```python
from build123d import *

# Parameters (mm, degrees)
SKETCH_1_W                = 38
SKETCH_1_H                = 46.5
EXTRUDE_1_DEPTH           = 7
SKETCH_2_W                = 5
SKETCH_2_H                = 38.5
CUT_EXTRUDE_1_DEPTH       = 52.100391388
SKETCH_3_W                = 7
SKETCH_3_H                = 39.5
CUT_EXTRUDE_2_DEPTH       = 52.100391388
SKETCH_4_W                = 7.5
SKETCH_4_H                = 20
CUT_EXTRUDE_3_DEPTH       = 52.100391388
SKETCH_5_W                = 7.5
SKETCH_5_H                = 20
CUT_EXTRUDE_4_DEPTH       = 52.100391388
SKETCH_6_W                = 26
SKETCH_6_H                = 6
EXTRUDE_2_DEPTH           = 41.75
HOLE_WIZARD_3_0_3_1_D     = 3
HOLE_WIZARD_3_0_3_1_DEPTH = 8
HOLE_WIZARD_3_0_3_2_D     = 3
HOLE_WIZARD_3_0_3_2_DEPTH = 48.75
HOLE_WIZARD_3_0_3_3_D     = 3
HOLE_WIZARD_M201_D        = 22.1
HOLE_WIZARD_M201_DEPTH    = 46.5
FILLET_1_R                = 10


with BuildPart() as part:
    # Эскиз1 → Бобышка-Вытянуть1 (new body)
    with BuildSketch(Plane(origin=(24.375, 0, 0), x_dir=(0, 0, -1), z_dir=(1, 0, 0))):
        with Locations((-1, 23.25)):
            Rectangle(SKETCH_1_W, SKETCH_1_H)
    extrude(amount=-EXTRUDE_1_DEPTH)

    # Эскиз2 → Вырез-Вытянуть1 (cut, through all)
    with BuildSketch(Plane.ZY.offset(-17.375)):
        with Locations((-15.5, 27.25)):
            Rectangle(SKETCH_2_W, SKETCH_2_H)
    extrude(amount=-CUT_EXTRUDE_1_DEPTH, mode=Mode.SUBTRACT)

    # Эскиз3 → Вырез-Вытянуть2 (cut, through all)
    with BuildSketch(Plane.ZY.offset(-17.375)):
        with Locations((16.5, 26.75)):
            Rectangle(SKETCH_3_W, SKETCH_3_H)
    extrude(amount=-CUT_EXTRUDE_2_DEPTH, mode=Mode.SUBTRACT)

    # Эскиз4 → Вырез-Вытянуть3 (cut, through all)
    with BuildSketch(Plane(origin=(24.375, 0, 0), x_dir=(0, 0, -1), z_dir=(1, 0, 0))):
        with Locations((-7.5, 28.5)):
            Rectangle(SKETCH_4_W, SKETCH_4_H)
    extrude(amount=-CUT_EXTRUDE_3_DEPTH, mode=Mode.SUBTRACT)

    # Эскиз5 → Вырез-Вытянуть4 (cut, through all)
    with BuildSketch(Plane.ZY.offset(-17.375)):
        with Locations((-7.5, 28.5)):
            Rectangle(SKETCH_5_W, SKETCH_5_H)
    extrude(amount=-CUT_EXTRUDE_4_DEPTH, mode=Mode.SUBTRACT)

    # Эскиз6 → Бобышка-Вытянуть2 (add)
    with BuildSketch(Plane.ZY.offset(-17.375)):
        with Locations((0, 3)):
            Rectangle(SKETCH_6_W, SKETCH_6_H)
    extrude(amount=EXTRUDE_2_DEPTH)

    # Диаметр отверстия Ø3.0 (3)1
    with Locations(Plane(origin=(0, 46.5, 0), x_dir=(1, 0, 0), z_dir=(0, 1, 0))):
        with Locations((20.875, -7.5), (20.875, 7.5)):
            Hole(HOLE_WIZARD_3_0_3_1_D / 2, depth=HOLE_WIZARD_3_0_3_1_DEPTH)

    # Диаметр отверстия Ø3.0 (3)2
    with Locations(Plane(origin=(24.375, 0, 0), x_dir=(0, 0, -1), z_dir=(1, 0, 0))):
        with Locations((-16.5, 3.5)):
            Hole(HOLE_WIZARD_3_0_3_2_D / 2, depth=HOLE_WIZARD_3_0_3_2_DEPTH)

    # Диаметр отверстия Ø3.0 (3)3 (through all)
    with Locations(Plane(origin=(0, 8, 0), x_dir=(1, 0, 0), z_dir=(0, 1, 0))):
        with Locations((20.875, 15.8)):
            Hole(HOLE_WIZARD_3_0_3_3_D / 2)

    # Отверстие с зазором M201
    with Locations(Plane(origin=(0, 0, 0), x_dir=(-1, 0, 0), z_dir=(0, -1, 0))):
        with Locations((11.375, 0)):
            Hole(HOLE_WIZARD_M201_D / 2, depth=HOLE_WIZARD_M201_DEPTH)

    # Скругление1
    fillet_1_edges = [part.edges().sort_by_distance(p)[0] for p in [
        (-24.375, 3, -13),
        (-24.375, 3, 13),
    ]]
    fillet(fillet_1_edges, radius=FILLET_1_R)


solid = part.part
```
Input: part model. Units: mm. Frame: model coordinates. A direction names the side the tool comes from. Give positions to 0.01 mm unless a question says otherwise; leave off trailing zeros. Order: outer loops, then holes, each group sorted by start corner. A loop starts at its lowest first (then second) coordinate and runs counter-clockwise, first axis right, second up. Notation, with made-up numbers: M -16.75,68 L 2.25,68 A6 ccw 2.25,72 Z; hole C -31,-3.75 d6. An arc over 180 degrees is marked long. Return JSON: item names as keys, results as strings.
1) Access query for faces 1 (the face through (2, 3, -13)), 2 (the face through (21, 27, -13)), 3 (the face through (21, 7, 16)). Directions: +Z, -Z, +X, -X, +Y, -Y. A direction counts if a zero-diameter tool reaches every point of the face in a straight line with its end or side. Return the directions, or none.
Taken from the geometry:
{"face 1": "-Z, -X, +Y, -Y", "face 2": "-Z, +X, -X, +Y", "face 3": "+Z, +X, -X, +Y"}
2) Section query A-A on z = 0. Output: boundary loops of the cut face in (x, y) (3 decimals), and give its area (3 significant figures).
Taken from the geometry:
{"outline": "M -24.375,0 L -22.425,0 L -22.425,6 L -24.375,6 Z; M -0.325,0 L 24.375,0 L 24.375,46.5 L 17.375,46.5 L 17.375,6 L -0.325,6 Z", "area": "443 mm2"}
3) Contact query for flat-ended pins moving along their axis: pin 1 (6 mm diameter, centred on x = -3.5, y = 8.5, fed in from +Z); pin 2 (4 mm diameter, centred on x = 3.5, z = -4.5, fed in from -Y); pin 3 (1.5 mm diameter, centred on x = 19.5, z = -15, fed in from +Y); pin 4 (10 mm diameter, centred on x = 8.5, z = 4.5, fed in from +Y). Output: stop coordinate, or through.
Taken from the geometry:
{"pin 1": "stops at z = 13", "pin 2": "stops at y = 0", "pin 3": "stops at y = 8", "pin 4": "stops at y = 6"}
4) Mould query, pull axis Z, two halves, no side actions, for faces 4 (the face through (-21.368, 3.042, 10.148)), 5 (the face through (17.375, 24, -3)), 6 (the face through (21, 28, 3.75)), 7 (the face through (22.065, 42.444, 8.413)). Classes: released by +Z, released by -Z, zero draft, split by the parting line, or undercut.
Taken from the geometry:
{"face 4": "released by +Z", "face 5": "zero draft", "face 6": "undercut", "face 7": "undercut"}
5) Section query C-C on x = -8. Output: boundary loops of the cut face in (y, z), and give its area (3 significant figures).
Taken from the geometry:
{"outline": "M 0,-13 L 6,-13 L 6,-10.52 L 0,-10.52 Z; M 0,10.52 L 6,10.52 L 6,13 L 0,13 Z", "area": "29.7 mm2"}
6) Section query B-B on y = 24. Output: boundary loops of the cut face in (x, z) (3 decimals), and give its area (3 significant figures).
Taken from the geometry:
{"outline": "M 17.375,-13 L 24.375,-13 L 24.375,-11.25 L 17.375,-11.25 Z; M 17.375,-3.75 L 24.375,-3.75 L 24.375,3.75 L 17.375,3.75 Z; M 17.375,11.25 L 24.375,11.25 L 24.375,13 L 17.375,13 Z", "area": "77.0 mm2"}
7) Line query: L1, parallel to Z at x = 22.5, y = 27; L2, parallel to Y at x = 19, z = 16.5; L3, parallel to Y at x = -22, z = -7.5. Output: solid intervals per line, ascending. Write a range as [from, to].
Taken from the geometry:
{"L1": "z = [-13, -11.25], [-3.75, 3.75], [11.25, 13]", "L2": "y = [0, 2], [5, 7]", "L3": "y = [0, 6]"}
8) Section query D-D on y = 42. Output: boundary loops of the cut face in (x, z) (3 decimals), and give its area (3 significant figures).
Taken from the geometry:
{"outline": "M 17.375,-13 L 24.375,-13 L 24.375,13 L 17.375,13 Z; hole C 20.875,-7.5 d3; hole C 20.875,7.5 d3", "area": "168 mm2"}
